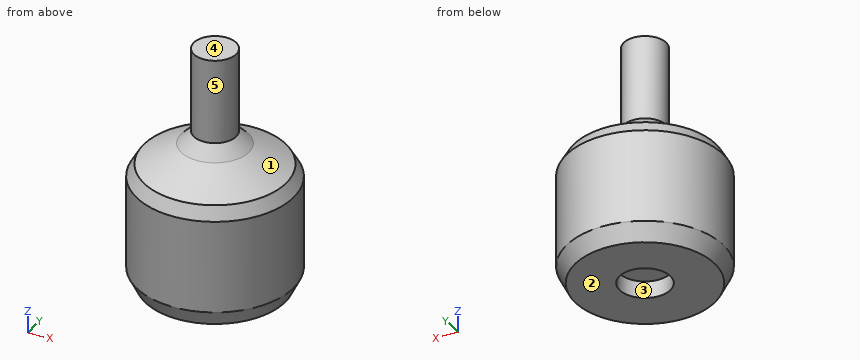
from build123d import *

# Parameters (mm, degrees)
F5_R       = 8.25
F6_R       = 9.25
F11_FACE_R = 9.25
F7_R       = 9.25
F12_FACE_R = 9.25
F9_R       = 4
F13_FACE_R = 4
F8_R       = 2.5
F14_FACE_R = 2.5
F10_R      = 2.5
F16_SIZE   = 1
F17_R      = 3
F18_DEPTH  = 2


with BuildPart() as f11:
    # F5 (on Top) → F11 section 0
    with BuildSketch(Plane.XY):
        Circle(F5_R)
    # F6 (on offset) → F11 section 1
    with BuildSketch(Plane.XY.offset(2)):
        Circle(F6_R)
    loft()

    # F11_face (on face) → F12 section 0
    with BuildSketch(Plane.XY.offset(2)):
        Circle(F11_FACE_R)
    # F7 (on offset) → F12 section 1
    with BuildSketch(Plane.XY.offset(14)):
        Circle(F7_R)
    loft()

    # F12_face (on face) → F13 section 0
    with BuildSketch(Plane.XY.offset(14)):
        Circle(F12_FACE_R)
    # F9 (on offset) → F13 section 1
    with BuildSketch(Plane.XY.offset(17)):
        Circle(F9_R)
    loft()

    # F13_face (on face) → F14 section 0
    with BuildSketch(Plane.XY.offset(17)):
        Circle(F13_FACE_R)
    # F8 (on offset) → F14 section 1
    with BuildSketch(Plane.XY.offset(18.5)):
        Circle(F8_R)
    loft()

    # F14_face (on face) → F15 section 0
    with BuildSketch(Plane.XY.offset(18.5)):
        Circle(F14_FACE_R)
    # F10 (on offset) → F15 section 1
    with BuildSketch(Plane.XY.offset(28.5)):
        Circle(F10_R)
    loft()

    # F16
    f16_edges = [f11.edges().sort_by_distance(p)[0] for p in [
        (-9.25, 0, 14),
    ]]
    chamfer(f16_edges, length=F16_SIZE)

    # F17 (on Top) → F18 (cut)
    with BuildSketch(Plane.XY):
        Circle(F17_R)
    extrude(amount=F18_DEPTH, mode=Mode.SUBTRACT)


solid = f11.part
Part model, mm, in its own coordinate system. Face numbers are marked on the shaded views. A direction names the side the tool comes from. Coordinates: 2 decimals unless noted, no trailing zeros. Order: outer loops, then holes, each group sorted by start corner. A loop starts at its lowest first (then second) coordinate and runs counter-clockwise, first axis right, second up. Notation, with made-up numbers: M -26.5,41 L -0.5,41 A16 cw -0.5,57 Z; hole C 78,21 d4. An arc over 180 degrees is marked long. Use a Markdown table: item, result.
(1) Pull direction Y, two halves, no side cores. Call the marked faces 1, 2 and 3: released by +Y, released by -Y, zero draft, split by the parting line, or undercut.
A:
| item | result |
|---|---|
| face 1 | split by the parting line |
| face 2 | zero draft |
| face 3 | undercut |
(2) Cut at A-A on z = 21.25. Write the cut outline in (x, y), then the cut area to 3 significant figures.
A:
| item | result |
|---|---|
| outline | C 0,0 d5 |
| area | 19.6 mm^2 |
(3) Flat gauge pins, fed straight in: pin 1 (2 mm diameter, centred on y = -1.5, z = 11, fed in from -X); pin 2 (6 mm diameter, centred on y = 4.5, z = 18, fed in from -X); pin 3 (3.5 mm diameter, centred on x = 0, y = 0, fed in from -Z). Where does each tip first touch, or does it go through?
A:
| item | result |
|---|---|
| pin 1 | stops at x = -9.24 |
| pin 2 | stops at x = -6.3 |
| pin 3 | stops at z = 2 |
(4) Cut at B-B on z = 5.75. Write the cut outline in (x, y), then the cut area to 3 significant figures.
A:
| item | result |
|---|---|
| outline | C 0,0 d18.5 |
| area | 269 mm^2 |
(5) Probe L1, parallel to Z at x = 0, y = 1.75; L2, parallel to Y at x = 0, z = 1.1; L3, parallel to Z at x = -3.75, y = -6.5. List the from-to ranges inside material, lowest first.
A:
| item | result |
|---|---|
| L1 | z = 2 to 28.5 |
| L2 | y = -8.8 to -3, 3 to 8.8 |
| L3 | z = 0 to 15 |
(6) Tool access for the marked faces 4 and 5: list every direction of +Z, -Z, +X, -X, +Y, -Y with a clear straight run to the whole face (end or side of a thin tool).
A:
| item | result |
|---|---|
| face 4 | +Z, +X, -X, +Y, -Y |
| face 5 | +Z |
